```python
from build123d import *

# Parameters (mm, degrees)
SKETCH1_R           = 4
BOSS_EXTRUDE1_DEPTH = 3


with BuildPart() as part:
    # Sketch1 → Boss-Extrude1 (new body)
    with BuildSketch(Plane.XY):
        Polygon((195.645, 0), (195.645, 37.18), (232.325, 37.18), (232.325, 192.825), (195.645, 192.825), (195.645, 196), (46.835, 196), (46.835, 180.82), (12.005, 180.82), (12.005, 145.99), (-3.175, 145.99), (-3.175, 34.005), (0, 34.005), (0, 0), align=None)
        with Locations((170.815, 19.005)):
            Circle(SKETCH1_R, mode=Mode.SUBTRACT)
        with Locations((24.83, 19.005)):
            Circle(SKETCH1_R, mode=Mode.SUBTRACT)
        with Locations((213.82, 62.01)):
            Circle(SKETCH1_R, mode=Mode.SUBTRACT)
        with Locations((213.82, 167.995)):
            Circle(SKETCH1_R, mode=Mode.SUBTRACT)
    extrude(amount=BOSS_EXTRUDE1_DEPTH)


solid = part.part
```
CAD build for the part. Positions are in the model's coordinates, mm. Give positions to 0.01 mm unless a question says otherwise; leave off trailing zeros. Loops run counter-clockwise (first coordinate to the right, second up) from the corner with the lowest first, then second, coordinate; pieces in that order, holes last. Notation, with made-up numbers: M 11.5,19.5 L 53.5,19.5 A21 cw 53.5,29.5 Z; hole C -26.75,7 d8. An arc over 180 degrees is marked long. Use one line per item in the form item = value.
Item 1: Slice it at C-C (x = 24.83). List the corners of the cut face in (y, z) (3 decimals).
Determined:
outline = M 0,0 L 15.005,0 L 15.005,3 L 0,3 Z; M 23.005,0 L 180.82,0 L 180.82,3 L 23.005,3 Z
Item 2: Slice it at A-A (y = 62.01). List the corners of the cut face in (x, z) (3 decimals), plus the area to 4 significant figures.
Determined:
outline = M -3.175,0 L 209.82,0 L 209.82,3 L -3.175,3 Z; M 217.82,0 L 232.325,0 L 232.325,3 L 217.82,3 Z
area = 682.5 mm2
Item 3: Slice it at D-D (z = 2.5). List the corners of the cut face in (x, y) (3 decimals), plus the area to 3 significant figures.
Determined:
outline = M -3.175,34.005 L 0,34.005 L 0,0 L 195.645,0 L 195.645,37.18 L 232.325,37.18 L 232.325,192.825 L 195.645,192.825 L 195.645,196 L 46.835,196 L 46.835,180.82 L 12.005,180.82 L 12.005,145.99 L -3.175,145.99 Z; hole C 24.83,19.005 d8; hole C 170.815,19.005 d8; hole C 213.82,62.01 d8; hole C 213.82,167.995 d8
area = 43,100 mm2
Item 4: Two-plate mould, pull along X, no slides. Class faces 1 (the face through (113, 99, 0)), 2 (the face through (174.63, 20.21, 1.48)): pulls with the +X half, pulls with the -X half, needs draft (parallel to the pull), parting line crosses it, or undercut.
Determined:
face_1 = needs draft
face_2 = undercut
Item 5: Flat gauge pins, fed straight in: pin 1 (0.9 mm diameter, centred on x = 208.5, z = 1.5, fed in from +Y) (3 decimals); pin 2 (0.9 mm diameter, centred on x = 5, z = 1.5, fed in from +Y); pin 3 (1.5 mm diameter, centred on y = 169, z = 2, fed in from -X) (3 decimals). Where does each tip first touch, or does it go through?
Determined:
pin_1 = 192.825
pin_2 = 145.99
pin_3 = 12.005
Item 6: Drill centre lines: probe 1 along Y at (x, z) = (213.82, 2.15) (3 decimals); probe 2 along Y at (x, z) = (25.5, 2.85); probe 3 along X at (y, z) = (8, 1.75) (3 decimals). Where is each one in solid material? Low to high. Write a range as from..to.
Determined:
probe_1 = 37.18..58.01, 66.01..163.995, 171.995..192.825
probe_2 = 0..15.06, 22.95..180.82
probe_3 = 0..195.645
Item 7: Slice it at B-B (x = 213.82). List the corners of the cut face in (y, z) (3 decimals).
Determined:
outline = M 37.18,0 L 58.01,0 L 58.01,3 L 37.18,3 Z; M 66.01,0 L 163.995,0 L 163.995,3 L 66.01,3 Z; M 171.995,0 L 192.825,0 L 192.825,3 L 171.995,3 Z
